Geometry check sheet. Reference: drawing and pictorial views, mm from the part's lowest x, y, z. Give positions to 0.01 mm unless a question says otherwise; leave off trailing zeros. Loops run counter-clockwise (first coordinate to the right, second up) from the corner with the lowest first, then second, coordinate; pieces in that order, holes last. Notation, with made-up numbers: (89.25, -8) - (142.25, -8) arc R20 ccw to (142.25, 12) - close; hole circle Ø1 at (18, -3.75). An arc over 180 degrees is marked (long way). Use CSV: the item, a comma, the result in double quotes.
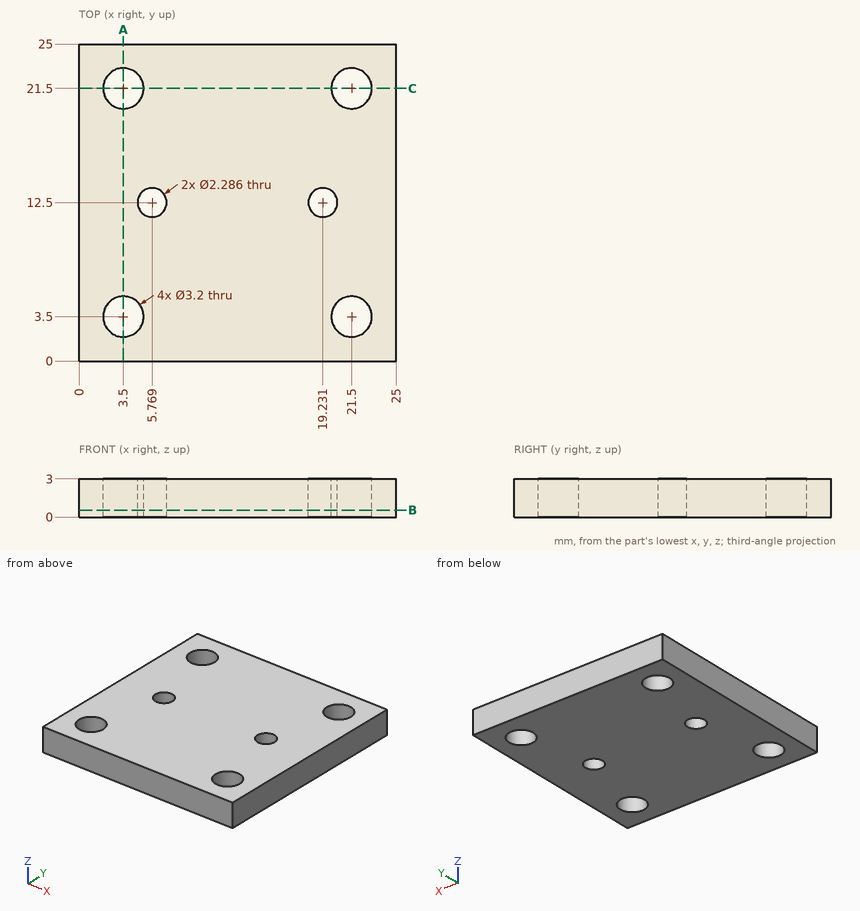
1. Sectioned sample at A-A, the plane x = 3.5. Record the boundary of the cut face in (y, z).
Completed:
outline,"(0, 0) - (1.9, 0) - (1.9, 3) - (0, 3) - close; (5.1, 0) - (19.9, 0) - (19.9, 3) - (5.1, 3) - close; (23.1, 0) - (25, 0) - (25, 3) - (23.1, 3) - close"
2. Go/stop test with a flat-tipped pin: pin 1 Ø1.5 at (x, z) = (12, 2.5) entering from -Y. Record where the tip stops, or that it passes through.
Completed:
pin 1,"stops at y = 0"
3. Sectioned sample at B-B, the plane z = 0.55. Record the boundary of the cut face in (x, y), and give its area (3 significant figures).
Completed:
outline,"(0, 0) - (25, 0) - (25, 25) - (0, 25) - close; hole circle Ø3.2 at (3.5, 3.5); hole circle Ø3.2 at (3.5, 21.5); hole circle Ø2.29 at (5.77, 12.5); hole circle Ø2.29 at (19.23, 12.5); hole circle Ø3.2 at (21.5, 3.5); hole circle Ø3.2 at (21.5, 21.5)"
area,"585 mm²"
4. Scan lines: line 1 along X through (y, z) = (12.5, 2.15); line 2 along Y through (x, z) = (21.5, 1.1). Record each from-to range of solid material in increasing order.
Completed:
line 1,"x = 0 to 4.63, 6.91 to 18.09, 20.37 to 25"
line 2,"y = 0 to 1.9, 5.1 to 19.9, 23.1 to 25"
